Verification items for the finished model (mm, model axes). Round coordinates to 2 decimals unless told otherwise and drop trailing zeros. Write each loop counter-clockwise with the first axis right and the second up, starting at its lowest first coordinate (ties: lowest second). Pieces come first, ordered by that corner, then holes. Notation, with made-up numbers: M 64,63 L 107,63 A22 cw 107,100 Z; hole C -26.75,-28.5 d7. An arc over 180 degrees is marked long. Write each question's results on one line, items separated by ' | '.
from build123d import *

# Parameters (mm, degrees)
SKETCH_1_W      = 40
SKETCH_1_H      = 40
SKETCH_1_R      = 1.5
EXTRUDE_1_DEPTH = 10
FILLET_1_R      = 5


with BuildPart() as part:
    # 草图1 → 凸台-拉伸1 (new body)
    with BuildSketch(Plane.XY):
        Rectangle(SKETCH_1_W, SKETCH_1_H)
        with Locations((-15, 15)):
            Circle(SKETCH_1_R, mode=Mode.SUBTRACT)
        with Locations((15, 15)):
            Circle(SKETCH_1_R, mode=Mode.SUBTRACT)
        with Locations((-15, -15)):
            Circle(SKETCH_1_R, mode=Mode.SUBTRACT)
        with Locations((15, -15)):
            Circle(SKETCH_1_R, mode=Mode.SUBTRACT)
    extrude(amount=EXTRUDE_1_DEPTH)

    # 圆角1
    fillet_1_edges = [part.edges().sort_by_distance(p)[0] for p in [
        (20, -20, 5),
        (-20, -20, 5),
        (-20, 20, 5),
        (20, 20, 5),
    ]]
    fillet(fillet_1_edges, radius=FILLET_1_R)


solid = part.part
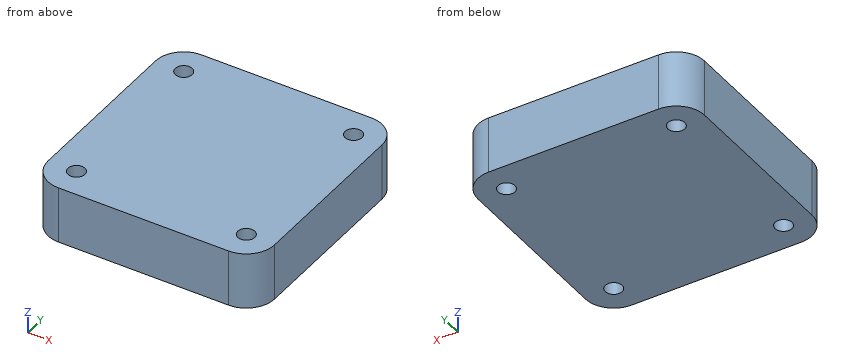
1) Depth check by flat-ended pin: P1, Ø1, axis at x = 2.5, y = 13.5, coming from the -Z side; P2, Ø1.8, axis at x = 15, y = -15, coming from the +Z side. Enter the tip coordinate at first touch or a pass-through.
Calculated:
P1: stops at z = 0 | P2: passes through
2) Material ranges on line 1 (Y direction, x = -15, z = 7.25); line 2 (Y direction, x = 15.5, z = 2); line 3 (X direction, y = -18, z = 2.25), recorded low to high. Write a range as [from, to].
Calculated:
line 1: y = [-20, -16.5], [-13.5, 13.5], [16.5, 20] | line 2: y = [-19.97, -16.41], [-13.59, 13.59], [16.41, 19.97] | line 3: x = [-19, 19]
3) Sectioned sample at A-A, the plane z = 4. Record the cut outline in (x, y).
Calculated:
outline: M -20,-15 A5 ccw -15,-20 L 15,-20 A5 ccw 20,-15 L 20,15 A5 ccw 15,20 L -15,20 A5 ccw -20,15 Z; hole C -15,-15 d3; hole C -15,15 d3; hole C 15,-15 d3; hole C 15,15 d3
4) Sectioned sample at B-B, the plane x = 14. Record the cut outline in (y, z).
Calculated:
outline: M -20,0 L -16.12,0 L -16.12,10 L -20,10 Z; M -13.88,0 L 13.88,0 L 13.88,10 L -13.88,10 Z; M 16.12,0 L 20,0 L 20,10 L 16.12,10 Z
